from build123d import *

# Parameters (mm, degrees)
SKETCH1_R           = 4.7625
BOSS_EXTRUDE1_DEPTH = 12.7
CHAMFER1_SIZE       = 0.254
SKETCH2_W           = 12.7
SKETCH2_H           = 12.7
BOSS_EXTRUDE2_DEPTH = 12.7
FILLET1_R           = 0.635
CUT_EXTRUDE2_START  = -20.32
SKETCH5_R           = 3.175
CUT_EXTRUDE2_DEPTH  = 20.32
SKETCH6_R           = 2.54
CUT_EXTRUDE3_DEPTH  = 23.876


with BuildPart() as part:
    # Sketch1 → Boss-Extrude1 (new body)
    with BuildSketch(Plane.XY):
        Circle(SKETCH1_R)
    extrude(amount=BOSS_EXTRUDE1_DEPTH)

    # Chamfer1
    chamfer1_edges = [part.edges().sort_by_distance(p)[0] for p in [
        (-4.7625, 0, 0),
    ]]
    chamfer(chamfer1_edges, length=CHAMFER1_SIZE)

    # Sketch2 → Boss-Extrude2 (add)
    with BuildSketch(Plane.XY.offset(12.7)):
        Rectangle(SKETCH2_W, SKETCH2_H)
    extrude(amount=BOSS_EXTRUDE2_DEPTH)

    # Sketch3 → Revolve1 (revolve)
    with BuildSketch(Plane(origin=(0, 0, 0), x_dir=(0, 0, -1), z_dir=(1, 0, 0))):
        Polygon((-25.4, 3.175), (-28.575, 3.175), (-28.575, 3.81), (-33.655, 3.175), (-33.655, 3.81), (-38.735, 3.175), (-38.735, 3.81), (-43.815, 3.175), (-43.815, 0), (-25.4, 0), align=None)
    revolve(axis=Axis((0, 0, 19.05), (0, 0, 1)))

    # Fillet1
    fillet1_edges = [part.edges().sort_by_distance(p)[0] for p in [
        (0, -3.175, 25.4),
        (-4.7625, 0, 12.7),
    ]]
    fillet(fillet1_edges, radius=FILLET1_R)

    # Sketch5 → Cut-Extrude2 (cut)
    with BuildSketch(Plane(origin=(0, 0, 0), x_dir=(-1, 0, 0), z_dir=(0, 0, -1)).offset(CUT_EXTRUDE2_START)):
        with Locations(Location((0, 0, 0), (0, 0, 90))):
            Circle(SKETCH5_R)
    extrude(amount=CUT_EXTRUDE2_DEPTH, mode=Mode.SUBTRACT)

    # Sketch6 → Cut-Extrude3 (cut)
    with BuildSketch(Plane.XY.offset(43.815)):
        Circle(SKETCH6_R)
    extrude(amount=-CUT_EXTRUDE3_DEPTH, mode=Mode.SUBTRACT)


solid = part.part
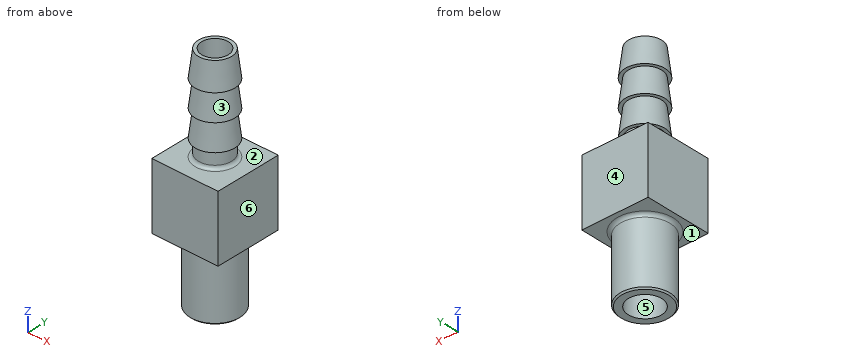
Verification items for the finished model (mm, model axes). Face numbers are marked on the shaded views. A direction names the side the tool comes from. Coordinates: 2 decimals unless noted, no trailing zeros. Order: outer loops, then holes, each group sorted by start corner. A loop starts at its lowest first (then second) coordinate and runs counter-clockwise, first axis right, second up.
Item 1: Section check B-B, the plane z = 36. Enter the section's corners in (x, y), then the cut area to 3 significant figures.
Filled in:
outline: circle Ø7.03 at (0, 0); hole circle Ø5.08 at (0, 0)
area: 18.6 mm2
Item 2: Section check A-A, the plane z = 16.5. Enter the section's corners in (x, y) (3 decimals), then the cut area to 3 significant figures.
Filled in:
outline: (-6.35, -6.35) - (6.35, -6.35) - (6.35, 6.35) - (-6.35, 6.35) - close; hole circle Ø6.35 at (0, 0)
area: 130 mm2
Item 3: Access from +Z, -Z, +X, -X, +Y, -Y to the whole of each face (thin tool, end or side, straight path). Record for the marked faces 1, 2 and 3.
Filled in:
face 1: -Z
face 2: +Z
face 3: none
Item 4: Material ranges on L1, parallel to X at y = 0, z = 14.75 (3 decimals); L2, parallel to Z at x = -5.5, y = -2.75; L3, parallel to Z at x = 1.75, y = 2.5 (3 decimals), recorded low to high.
Filled in:
L1: x = -6.35 to -3.175, 3.175 to 6.35
L2: z = 12.7 to 25.4
L3: z = 20.32 to 43.815
Item 5: Depth check by flat-ended pin: pin 1 (3 mm diameter, centred on x = -1, y = 1.5, fed in from +Z) (3 decimals); pin 2 (4 mm diameter, centred on x = 0, y = -0.5, fed in from -Z) (3 decimals); pin 3 (4 mm diameter, centred on x = -4.5, z = 35.5, fed in from +Y). Enter the tip coordinate at first touch or a pass-through.
Filled in:
pin 1: stops at z = 43.815
pin 2: passes through
pin 3: stops at y = 2.59
Item 6: Release check for a two-part mould opening along Y. For the marked faces 4, 5 and 6 record: +Y half, -Y half, draft (parallel to the pull), parting line (faces both ways), or undercut.
Filled in:
face 4: +Y half
face 5: undercut
face 6: draft
